Read the model definition and answer for the solid it produces. Units are mm, in the model's axes. Face numbers are marked on the shaded views. A direction names the side the tool comes from. Coordinates: 2 decimals unless noted, no trailing zeros. Loops run counter-clockwise (first coordinate to the right, second up) from the corner with the lowest first, then second, coordinate; pieces in that order, holes last.
Q1. Section D-D (y = 209) is taken. Give the vertices of the cut face in (x, z) (3 decimals).
Q2. Section A-A (y = 263.5) is taken. Give the vertices of the cut face in (x, z) (3 decimals).
Q3. Which of the six approach directions +Z, -Z, +X, -X, +Y, -Y give full straight-line access (tool end or side, diameter ignored) to the marked faces 1 and 2?
Q4. Section C-C (x = -133.5) is taken. Give the vertices of the cut face in (y, z) (3 decimals), then the cut area to 3 significant figures.
Q5. Straight lines are drawn through the part: line 1 (Z direction, x = -119.5, y = 44); line 2 (X direction, y = 65, z = -29); line 3 (Z direction, x = -76.5, y = 288). For each, find the intervals that lie inside material, in ascending order.
Q6. Flat-ended cylindrical pins translate along their axes: P1, Ø6.5, axis at x = 388.5, z = 15, coming from the -Y side; P2, Ø2, axis at x = -206, y = 155, coming from the -Z side; P3, Ø10, axis at y = 143, z = 178.5, coming from the +X side. Find the tip coordinate at first contact, or state that the pin passes through.
Q7. Section B-B (z = 30) is taken. Give the vertices of the cut face in (x, y) (3 decimals).
Autodesk Inventor part; units mm, degrees
ref_plane "YZ Plane" through (0, 0, 0) normal (1, 0, 0) x (0, 1, 0)
ref_plane "XZ Plane" through (0, 0, 0) normal (0, 1, 0) x (-1, 0, 0)
ref_plane "XY Plane" through (0, 0, 0) normal (0, 0, 1) x (1, 0, 0)
sketch "Sketch1" plane through (0, 0, 0) normal (0, 1, 0) x (-1, 0, 0)
  line L0 (381, 203.2) -> (-381, 203.2)
  line L1 (-381, 203.2) -> (-381, -203.2)
  line L2 (-381, -203.2) -> (381, -203.2)
  line L3 (381, -203.2) -> (381, 203.2)
  line L4 (381, 203.2) -> (-381, -203.2) construction
  line L5 (-381, 203.2) -> (381, -203.2) construction
  point P0 (0, 0)
  dimension "d0" = 762
  dimension "d1" = 406.4
extrude "Extrusion1" add sketch "Sketch1" along normal blind 311.15
sketch "Sketch2" plane through (0, 311.15, 0) normal (0, 1, 0) x (1, 0, 0)
  line L0 (-387.35, -209.55) -> (387.35, -209.55)
  line L1 (387.35, -209.55) -> (387.35, 209.55)
  line L2 (387.35, 209.55) -> (-387.35, 209.55)
  line L3 (-387.35, 209.55) -> (-387.35, -209.55)
  line L4 (-387.35, -209.55) -> (387.35, 209.55) construction
  line L5 (387.35, -209.55) -> (-387.35, 209.55) construction
  point P0 (-381, -203.2)
  point P1 (381, -203.2)
  point P2 (0, 0)
  dimension "d20" = 774.7
  dimension "d21" = 419.1
extrude "Extrusion2" add sketch "Sketch2" against normal blind 28.575
sketch "Sketch3" plane through (-381, 0, 203.2) normal (0, 0, 1) x (1, 0, 0)
  line L0 (358.775, 190.5) -> (403.225, 190.5)
  line L1 (403.225, 190.5) -> (403.225, 282.575)
  line L2 (403.225, 282.575) -> (358.775, 282.575)
  line L3 (358.775, 282.575) -> (358.775, 190.5)
  line L4 (762, 282.575) -> (0, 282.575) construction
  point P0 (381, 0)
  point P1 (381, 190.5)
  dimension "d7" = 44.45
  dimension "d8" = 190.5
extrude "Extrusion3" add sketch "Sketch3" along normal blind 25.4
sketch "Sketch4" plane through (381, 0, 203.2) normal (1, 0, 0) x (0, 0, -1)
  line L0 (152.4, 158.75) -> (254, 158.75)
  line L1 (254, 158.75) -> (254, 234.95)
  line L2 (254, 234.95) -> (152.4, 234.95)
  line L3 (152.4, 234.95) -> (152.4, 158.75)
  point P0 (203.2, 0)
  point P1 (203.2, 158.75)
  dimension "d11" = 101.6
  dimension "d12" = 158.75
  dimension "d13" = 76.2
extrude "Extrusion4" add sketch "Sketch4" along normal blind 12.7
mirror "Mirror1" about plane through (0, 0, 0) normal (1, 0, 0) of "Extrusion4"
properties part number "Jobox tool box" material "Copper"
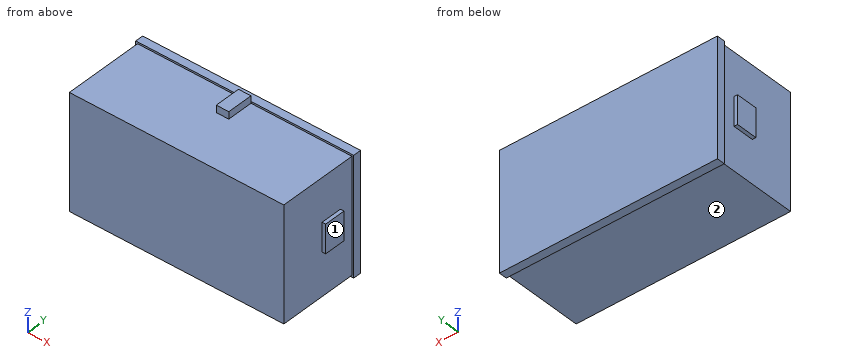
Numbers:
1. outline: (-393.7, -50.8) - (-381, -50.8) - (-381, -203.2) - (381, -203.2) - (381, -50.8) - (393.7, -50.8) - (393.7, 50.8) - (381, 50.8) - (381, 203.2) - (22.225, 203.2) - (22.225, 228.6) - (-22.225, 228.6) - (-22.225, 203.2) - (-381, 203.2) - (-381, 50.8) - (-393.7, 50.8) - close
2. outline: (-381, -203.2) - (381, -203.2) - (381, 203.2) - (22.225, 203.2) - (22.225, 228.6) - (-22.225, 228.6) - (-22.225, 203.2) - (-381, 203.2) - close
3. face 1: +Z, -Z, +X, +Y, -Y
3. face 2: -Z, +X, -X, -Y
4. outline: (0, -203.2) - (282.575, -203.2) - (282.575, -209.55) - (311.15, -209.55) - (311.15, 209.55) - (282.575, 209.55) - (282.575, 203.2) - (0, 203.2) - close
4. area: 127,000 mm2
5. line 1: z = -203.2 to 203.2
5. line 2: x = -381 to 381
5. line 3: z = -209.55 to 209.55
6. P1: stops at y = 158.75
6. P2: stops at z = -203.2
6. P3: stops at x = 381
7. outline: (-393.7, 158.75) - (-381, 158.75) - (-381, 0) - (381, 0) - (381, 158.75) - (393.7, 158.75) - (393.7, 234.95) - (381, 234.95) - (381, 282.575) - (387.35, 282.575) - (387.35, 311.15) - (-387.35, 311.15) - (-387.35, 282.575) - (-381, 282.575) - (-381, 234.95) - (-393.7, 234.95) - close
